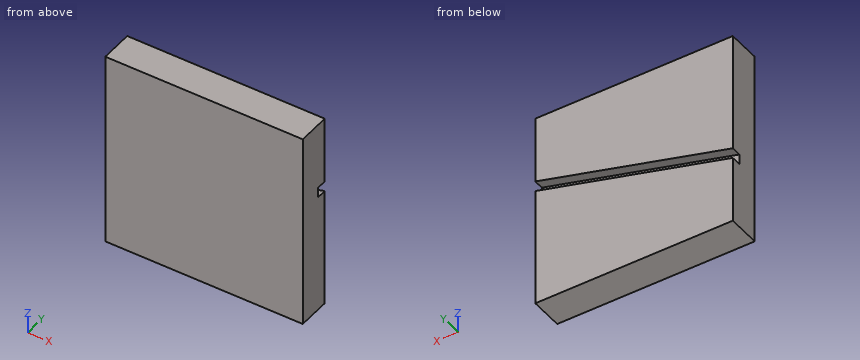
from build123d import *

# Parameters (mm, degrees)
SKETCH1_W           = 60
SKETCH1_H           = 60
BOSS_EXTRUDE1_DEPTH = 10
CUT_EXTRUDE1_DEPTH  = 3


with BuildPart() as part:
    # Sketch1 → Boss-Extrude1 (new body)
    with BuildSketch(Plane(origin=(0, 0, 0), x_dir=(1, 0, 0), z_dir=(0, 1, 0))):
        Rectangle(SKETCH1_W, SKETCH1_H)
    extrude(amount=BOSS_EXTRUDE1_DEPTH)

    # Sketch2 → Cut-Extrude1 (cut)
    with BuildSketch(Plane(origin=(0, 10, 0), x_dir=(1, 0, 0), z_dir=(0, 1, 0))):
        Polygon((-34.982332013, 7.820573342), (49.768078516, -14.888230718), (50.544535652, -11.990453239), (-34.205874878, 10.718350821), align=None)
    extrude(amount=-CUT_EXTRUDE1_DEPTH, mode=Mode.SUBTRACT)


solid = part.part
Source: CAD feature listing. Evaluate the final solid. Frame: model axes, mm. Give positions to 0.01 mm unless a question says otherwise; leave off trailing zeros. Order: outer loops, then holes, each group sorted by start corner. A loop starts at its lowest first (then second) coordinate and runs counter-clockwise, first axis right, second up. Notation, with made-up numbers: (57, 16) -> (75, 16) arc R16 cw to (75, 46) -> close; hole circle Ø7 at (14.25, 11). An arc over 180 degrees is marked (long way). Write item = value, one per line.
Q1. Cut plane C-C, the plane x = -13.5. Output: boundary loops of the cut face in (y, z).
Data:
outline = (0, -30) -> (10, -30) -> (10, -5.17) -> (7, -5.17) -> (7, -2.06) -> (10, -2.06) -> (10, 30) -> (0, 30) -> close
Q2. Cut plane A-A, the plane y = 9. Output: boundary loops of the cut face in (x, z), and give its area (3 significant figures).
Data:
outline = (-30, -30) -> (30, -30) -> (30, 6.49) -> (-30, -9.59) -> close; (-30, -6.49) -> (30, 9.59) -> (30, 30) -> (-30, 30) -> close
area = 3,410 mm^2
Q3. Cut plane B-B, the plane z = -3.5. Output: boundary loops of the cut face in (x, y), and give its area (3 significant figures).
Data:
outline = (-30, 0) -> (30, 0) -> (30, 10) -> (-7.27, 10) -> (-7.27, 7) -> (-18.86, 7) -> (-18.86, 10) -> (-30, 10) -> close
area = 565 mm^2
Q4. Material intervals for line 1 (Z direction, x = 13, y = 8.75); line 2 (Z direction, x = -26, y = 9); line 3 (Y direction, x = -0.5, z = 1), sorted ascending. Write a range as from..to.
Data:
line_1 = -30..1.93, 5.04..30
line_2 = -30..-8.52, -5.41..30
line_3 = 0..7
